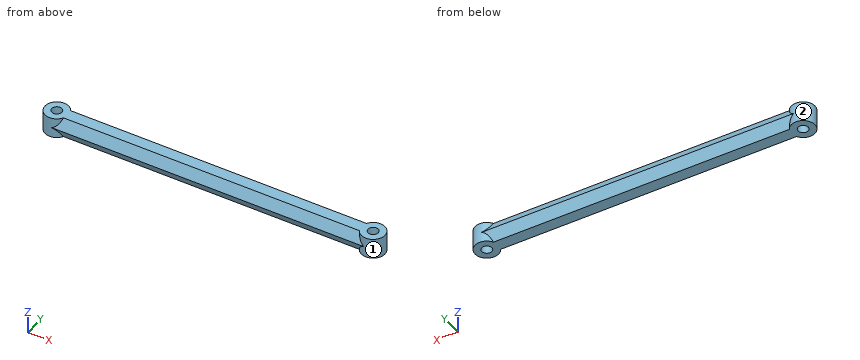
from build123d import *

# Parameters (mm, degrees)
SKETCH1_R                            = 3.5
SKETCH1_R_2                          = 1.5
BOSS_EXTRUDE1_DEPTH                  = 3
BOSS_EXTRUDE1_2_DEPTH                = 3
BOSS_EXTRUDE2_REACH                  = 52.71
BOSS_EXTRUDE2_END_RADIUS             = 3.5
BOSS_EXTRUDE2_DIRECTION_2_REACH      = 52.71
BOSS_EXTRUDE2_DIRECTION_2_END_RADIUS = 3.5


with BuildPart() as part:
    # Sketch1 → Boss-Extrude1 (new, symmetric)
    with BuildSketch(Plane.XY):
        with Locations((-47, 0)):
            Circle(SKETCH1_R)
        with Locations((-47, 0)):
            Circle(SKETCH1_R_2, mode=Mode.SUBTRACT)
    extrude(amount=BOSS_EXTRUDE1_DEPTH, both=True)



with BuildPart() as body_2:
    # Sketch1 → Boss-Extrude1 2 (new, symmetric)
    with BuildSketch(Plane.XY):
        with Locations((47, 0)):
            Circle(SKETCH1_R)
        with Locations((47, 0)):
            Circle(SKETCH1_R_2, mode=Mode.SUBTRACT)
    extrude(amount=BOSS_EXTRUDE1_2_DEPTH, both=True)


with BuildPart() as part_1:
    add(part.part)

    add(body_2.part)  # Boss-Extrude2 merges body 2
    # Boss-Extrude2: up to this cylinder (the profile starts outside it)
    boss_extrude2_end = Plane(origin=(-47, 0, 0), z_dir=(0, 0, -1)) * Cylinder(BOSS_EXTRUDE2_END_RADIUS, 113.42, mode=Mode.PRIVATE)
    # Sketch2 → Boss-Extrude2 (add, up to the surface)
    with BuildSketch(Plane(origin=(0, 0, 0), x_dir=(0, 0, -1), z_dir=(1, 0, 0)), mode=Mode.PRIVATE) as boss_extrude2_sk1:
        Polygon((-3, 1.732050808), (-3, -1.732050808), (0, -3.464101615), (3, -1.732050808), (3, 1.732050808), (0, 3.464101615), align=None)
    boss_extrude2_tool1 = extrude(boss_extrude2_sk1.sketch, amount=-BOSS_EXTRUDE2_REACH, mode=Mode.PRIVATE) - boss_extrude2_end
    add(boss_extrude2_tool1.solids().sort_by_distance((0, 0, 0))[0])

    # Boss-Extrude2 direction 2: up to this cylinder (the profile starts outside it)
    boss_extrude2_direction_2_end = Plane(origin=(47, 0, 0), z_dir=(0, 0, -1)) * Cylinder(BOSS_EXTRUDE2_DIRECTION_2_END_RADIUS, 113.42, mode=Mode.PRIVATE)
    # Sketch2 → Boss-Extrude2 direction 2 (add, up to the surface)
    with BuildSketch(Plane(origin=(0, 0, 0), x_dir=(0, 0, -1), z_dir=(1, 0, 0)), mode=Mode.PRIVATE) as boss_extrude2_direction_2_sk1:
        Polygon((-3, 1.732050808), (-3, -1.732050808), (0, -3.464101615), (3, -1.732050808), (3, 1.732050808), (0, 3.464101615), align=None)
    boss_extrude2_direction_2_tool1 = extrude(boss_extrude2_direction_2_sk1.sketch, amount=BOSS_EXTRUDE2_DIRECTION_2_REACH, mode=Mode.PRIVATE) - boss_extrude2_direction_2_end
    add(boss_extrude2_direction_2_tool1.solids().sort_by_distance((0, 0, 0))[0])


solid = part_1.part
Source: CAD feature listing. Evaluate the final solid. Frame: model axes, mm. Face numbers are marked on the shaded views. Coordinates: 2 decimals unless noted, no trailing zeros. Loops run counter-clockwise (first coordinate to the right, second up) from the corner with the lowest first, then second, coordinate; pieces in that order, holes last. Notation, with made-up numbers: (13.25, 28.25) - (27.25, 28.25) arc R28 cw to (27.25, 66.25) - close; hole circle Ø5 at (24.25, -28.75). An arc over 180 degrees is marked (long way). One line per item, written item: value. Start each with the question number.
1. Ray query, L1, parallel to X at y = 0.25, z = 0; L2, parallel to X at y = -1, z = 1; L3, parallel to Y at x = -47, z = 1.55. Return the intervals inside material, ascending.
2. Section B-B (z = -2). Return the cut outline in (x, y), and give its area (3 significant figures).
3. Section A-A (x = 29.5). Return the cut outline in (y, z), and give its area (3 significant figures).
4. Mould query, pull axis X, two halves, no side actions, for the marked faces 1 and 2. Classes: pulls with the +X half, pulls with the -X half, needs draft (parallel to the pull), parting line crosses it, or undercut.
Verdict:
1. L1: x = -50.49 to -48.48, -45.52 to 45.52, 48.48 to 50.49
1. L2: x = -50.35 to -48.12, -45.88 to 45.88, 48.12 to 50.35
1. L3: y = -3.5 to -1.5, 1.5 to 3.5
2. outline: (-44.37, -2.31) - (44.37, -2.31) arc R3.5 ccw (long way) to (44.37, 2.31) - (-44.37, 2.31) arc R3.5 ccw (long way) to start; hole circle Ø3 at (-47, 0); hole circle Ø3 at (47, 0)
2. area: 467 mm2
3. outline: (-3.46, 0) - (-1.73, -3) - (1.73, -3) - (3.46, 0) - (1.73, 3) - (-1.73, 3) - close
3. area: 31.2 mm2
4. face 1: undercut
4. face 2: undercut
